The model under review builds one solid part; all positions refer to its coordinate system, in mm. Face numbers are marked on the shaded views. Round coordinates to 2 decimals unless told otherwise and drop trailing zeros. Order: outer loops, then holes, each group sorted by start corner. A loop starts at its lowest first (then second) coordinate and runs counter-clockwise, first axis right, second up. Notation, with made-up numbers: M 21,-8 L 27,-8 A16 cw 27,6 Z; hole C 24.5,19 d3. An arc over 180 degrees is marked long. Answer as a JSON object with one key per item and string values. Group by question number.
1. Clearance check with flat-ended pins moving along their axes: P1, Ø8, axis at y = 10, z = -8.5, coming from the +X side; P2, Ø1.5, axis at x = -28.5, y = 15.5, coming from the +Z side; P3, Ø10, axis at y = 20, z = -0.5, coming from the -X side; P4, Ø5, axis at y = 9.5, z = -14.5, coming from the +X side. State where each tip first meets the part, or that it passes through.
2. Mouldability with a two-part tool opening along X and no side actions: class the marked faces 1, 2 and 3 as released by +X, released by -X, zero draft, split by the parting line, or undercut.
3. Add section D-D on z = -10. State the section outline as (x, y) points.
4. Add section A-A on z = 0. State the section outline as (x, y) points.
5. Add section B-B on x = 4.5. State the section outline as (y, z) points, and give its area (3 significant figures).
6. To check wall thickness, follow probe 1 along X at (y, z) = (18, -0.5); probe 2 along Y at (x, z) = (-30.5, 17); probe 3 along Z at (x, y) = (54.5, 8). State the ranges of each line that lie inside material, in increasing order. Write a range as [from, to].
7. Add section C-C on y = 5.5. State the section outline as (x, z) points, and give its area (3 significant figures).
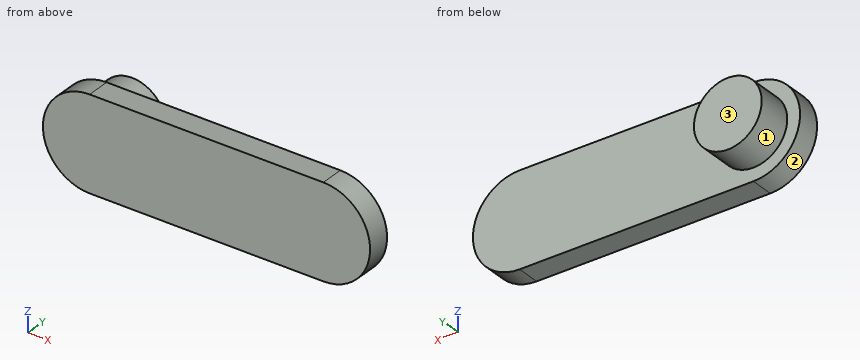
```python
from build123d import *

# Parameters (mm, degrees)
BOSS_EXTRUDE2_DEPTH = 10
SKETCH2_R           = 14.5
BOSS_EXTRUDE3_DEPTH = 15


with BuildPart() as part:
    # Sketch1 → Boss-Extrude2 (new body)
    with BuildSketch(Plane(origin=(0, 0, 0), x_dir=(1, 0, 0), z_dir=(0, 1, 0))):
        with BuildLine():
            Line((-45.740165089, 20), (54.259834911, 20))
            ThreePointArc((54.259834911, 20), (74.259834911, 0), (54.259834911, -20))
            Line((54.259834911, -20), (-45.740165089, -20))
            ThreePointArc((-45.740165089, -20), (-65.740165089, 0), (-45.740165089, 20))
        make_face()
    extrude(amount=BOSS_EXTRUDE2_DEPTH)

    # Sketch2 → Boss-Extrude3 (add)
    with BuildSketch(Plane(origin=(0, 10, 0), x_dir=(1, 0, 0), z_dir=(0, 1, 0))):
        with Locations(Location((-45.740165089, 0, 0), (0, 0, 270))):
            Circle(SKETCH2_R)
    extrude(amount=BOSS_EXTRUDE3_DEPTH)


solid = part.part
```
Recorded:
{
 "1": {"P1": "stops at x = 73.75", "P2": "passes through", "P3": "stops at x = -60.24", "P4": "stops at x = 70.26"},
 "2": {"face 1": "split by the parting line", "face 2": "released by -X", "face 3": "zero draft"},
 "3": {"outline": "M -63.06,0 L 71.58,0 L 71.58,10 L -35.24,10 L -35.24,25 L -56.24,25 L -56.24,10 L -63.06,10 Z"},
 "4": {"outline": "M -65.74,0 L 74.26,0 L 74.26,10 L -31.24,10 L -31.24,25 L -60.24,25 L -60.24,10 L -65.74,10 Z"},
 "5": {"outline": "M 0,-20 L 10,-20 L 10,20 L 0,20 Z", "area": "400 mm²"},
 "6": {"probe 1": "x = [-60.23, -31.25]", "probe 2": "y = [0, 10]", "probe 3": "z = [-20, 20]"},
 "7": {"outline": "M -45.74,-20 L 54.26,-20 A20 ccw 54.26,20 L -45.74,20 A20 ccw Z", "area": "5,260 mm²"}
}
